For this review, take the finished solid that the model builds, in its own axes (mm). A direction names the side the tool comes from. Round coordinates to 2 decimals unless told otherwise and drop trailing zeros. Write each loop counter-clockwise with the first axis right and the second up, starting at its lowest first coordinate (ties: lowest second). Pieces come first, ordered by that corner, then holes. Notation, with made-up numbers: (-0.75, -3.5) -> (26.25, -3.5) arc R16 cw to (26.25, 2.5) -> close; hole circle Ø9 at (56, 14.25). An arc over 180 degrees is marked (long way). Answer as CSV lines item,"result". Start each with the question number.
Item 1: Take a section at D-D on x = 12.7. Give the boundary of the cut face in (y, z), then the cut area to 3 significant figures.
Item 2: Take a section at A-A on x = -6. Give the boundary of the cut face in (y, z), then the cut area to 3 significant figures.
Item 3: Take a section at B-B on z = 0. Give the boundary of the cut face in (x, y).
Item 4: Take a section at C-C on y = 1. Give the boundary of the cut face in (x, z), then the cut area to 3 significant figures.
Item 5: Wall thickness on probe 1 along X at (y, z) = (0.5, 0); probe 2 along Z at (x, y) = (-6.5, 0.2); probe 3 along Z at (x, y) = (12.7, 1.65): over which ranges is each line inside the solid? List them lowest first. Write a range as from..to.
Item 6: Machinability: for faces 1 (the flat face through (8.9, 1, 3.1)), 2 (the flat face through (-5, 1, -1.403)), which of the approach directions +Z, -Z, +X, -X, +Y, -Y give a long, thin tool a straight path to every point of the face, cutting with its end or side? Answer none if there is none.
Item 7: For pin 1 Ø3 at (x, z) = (5.5, -1) entering from -Y, flat-tipped, find the tip position at first contact; note if it passes through.
Item 8: Mouldability with a two-part tool opening along Z and no side actions: class faces 3 (the flat face through (-5, 1, -3.658)), 4 (the cylindrical face through (-11.684, 1.03, 0.031)), 5 (the flat face through (-5, 1, 3.658)), 6 (the cylindrical face through (11.97, 1.03, -0.03)) as +Z half, -Z half, draft (parallel to the pull), parting line (faces both ways), or undercut.
```python
from build123d import *

# Parameters (mm, degrees)
BOSS_EXTRUDE1_DEPTH = 2.032
CUT_EXTRUDE1_REACH  = 4.032
CUT_EXTRUDE2_REACH  = 4.032
SKETCH3_R           = 0.73025


with BuildPart() as part:
    # Sketch1 → Boss-Extrude1 (new body)
    with BuildSketch(Plane(origin=(0, 0, 0), x_dir=(1, 0, 0), z_dir=(0, 1, 0))):
        with BuildLine():
            Line((-15.24, 3.6576), (-15.24, -3.6576))
            Line((-15.24, -3.6576), (4.953, -3.6576))
            Line((4.953, -3.6576), (13.054677298, -2.51511511))
            ThreePointArc((13.054677298, -2.51511511), (15.24, 0), (13.054677298, 2.51511511))
            Line((13.054677298, 2.51511511), (4.953, 3.6576))
            Line((4.953, 3.6576), (-15.24, 3.6576))
        make_face()
    extrude(amount=BOSS_EXTRUDE1_DEPTH)

    # Sketch2 → Cut-Extrude1 (cut, up to next)
    with BuildSketch(Plane(origin=(0, 2.032, 0), x_dir=(1, 0, 0), z_dir=(0, 1, 0)), mode=Mode.PRIVATE) as cut_extrude1_sk1:
        with BuildLine():
            Line((-10.28065, 1.40335), (-0.26035, 1.40335))
            ThreePointArc((-0.26035, 1.40335), (1.143, 0), (-0.26035, -1.40335))
            Line((-0.26035, -1.40335), (-10.28065, -1.40335))
            ThreePointArc((-10.28065, -1.40335), (-11.684, 0), (-10.28065, 1.40335))
        make_face()
    cut_extrude1_tool1 = extrude(cut_extrude1_sk1.sketch, amount=-CUT_EXTRUDE1_REACH, mode=Mode.PRIVATE) & part.part
    add(cut_extrude1_tool1.solids().sort_by_distance((-5.2705, 2.032, 0))[0], mode=Mode.SUBTRACT)

    # Sketch3 → Cut-Extrude2 (cut, up to next)
    with BuildSketch(Plane(origin=(0, 2.032, 0), x_dir=(1, 0, 0), z_dir=(0, 1, 0)), mode=Mode.PRIVATE) as cut_extrude2_sk1:
        with Locations((12.7, 0)):
            Circle(SKETCH3_R)
    cut_extrude2_tool1 = extrude(cut_extrude2_sk1.sketch, amount=-CUT_EXTRUDE2_REACH, mode=Mode.PRIVATE) & part.part
    add(cut_extrude2_tool1.solids().sort_by_distance((12.7, 2.032, 0))[0], mode=Mode.SUBTRACT)


solid = part.part
```
Output values:
1,outline,"(0, -2.57) -> (2.03, -2.57) -> (2.03, -0.73) -> (0, -0.73) -> close; (0, 0.73) -> (2.03, 0.73) -> (2.03, 2.57) -> (0, 2.57) -> close"
1,area,"7.46 mm^2"
2,outline,"(0, -3.66) -> (2.03, -3.66) -> (2.03, -1.4) -> (0, -1.4) -> close; (0, 1.4) -> (2.03, 1.4) -> (2.03, 3.66) -> (0, 3.66) -> close"
2,area,"9.16 mm^2"
3,outline,"(-15.24, 0) -> (-11.68, 0) -> (-11.68, 2.03) -> (-15.24, 2.03) -> close; (1.14, 0) -> (11.97, 0) -> (11.97, 2.03) -> (1.14, 2.03) -> close; (13.43, 0) -> (15.24, 0) -> (15.24, 2.03) -> (13.43, 2.03) -> close"
4,outline,"(-15.24, -3.66) -> (4.95, -3.66) -> (13.05, -2.52) arc R2.54 ccw to (13.05, 2.52) -> (4.95, 3.66) -> (-15.24, 3.66) -> close; hole (-10.28, -1.4) -> (-0.26, -1.4) arc R1.4 ccw to (-0.26, 1.4) -> (-10.28, 1.4) arc R1.4 ccw to start; hole circle Ø1.46 at (12.7, 0)"
4,area,"170 mm^2"
5,probe 1,"x = -15.24..-11.68, 1.14..11.97, 13.43..15.24"
5,probe 2,"z = -3.66..-1.4, 1.4..3.66"
5,probe 3,"z = -2.57..-0.73, 0.73..2.57"
6,face 1,"+Z, +X, +Y, -Y"
6,face 2,"+Y, -Y"
7,pin 1,"stops at y = 0"
8,face 3,"-Z half"
8,face 4,"undercut"
8,face 5,"+Z half"
8,face 6,"undercut"
